from build123d import *

# Parameters (mm, degrees)
SKETCH1_R           = 15
BOSS_EXTRUDE1_DEPTH = 10
SKETCH2_R           = 22.5
BOSS_EXTRUDE2_DEPTH = 8
CHAMFER1_SIZE       = 1
SKETCH3_R           = 10
CUT_EXTRUDE1_DEPTH  = 10
CUT_EXTRUDE2_DEPTH  = 3
CHAMFER2_SIZE       = 1


with BuildPart() as part:
    # Sketch1 → Boss-Extrude1 (new body)
    with BuildSketch(Plane(origin=(0, 0, 0), x_dir=(1, 0, 0), z_dir=(0, 1, 0))):
        with Locations(Location((0, 0, 0), (0, 0, 270))):
            Circle(SKETCH1_R)
    extrude(amount=BOSS_EXTRUDE1_DEPTH)

    # Sketch2 → Boss-Extrude2 (add)
    with BuildSketch(Plane(origin=(0, 10, 0), x_dir=(1, 0, 0), z_dir=(0, 1, 0))):
        with Locations(Location((0, 0, 0), (0, 0, 270))):
            Circle(SKETCH2_R)
    extrude(amount=BOSS_EXTRUDE2_DEPTH)

    # Chamfer1
    chamfer1_edges = [part.edges().sort_by_distance(p)[0] for p in [
        (0, 0, -15),
    ]]
    chamfer(chamfer1_edges, length=CHAMFER1_SIZE)

    # Sketch3 → Cut-Extrude1 (cut)
    with BuildSketch(Plane.XZ):
        with Locations(Location((0, 0, 0), (0, 0, 270))):
            Circle(SKETCH3_R)
    extrude(amount=-CUT_EXTRUDE1_DEPTH, mode=Mode.SUBTRACT)

    # Sketch4 → Cut-Extrude2 (cut)
    with BuildSketch(Plane(origin=(0, 18, 0), x_dir=(1, 0, 0), z_dir=(0, 1, 0))):
        Polygon((5.326189108, -2.228237625), (4.592804943, 3.49849626), (-0.733384165, 5.726733886), (-5.326189108, 2.228237625), (-4.592804943, -3.49849626), (0.733384165, -5.726733886), align=None)
    extrude(amount=-CUT_EXTRUDE2_DEPTH, mode=Mode.SUBTRACT)

    # Chamfer2
    chamfer2_edges = [part.edges().sort_by_distance(p)[0] for p in [
        (0, 0, 10),
    ]]
    chamfer(chamfer2_edges, length=CHAMFER2_SIZE)


solid = part.part
Check sheet for the modelled part. Datum: model origin and axes. Units: mm. A direction names the side the tool comes from. Coordinates: 2 decimals unless noted, no trailing zeros. Loops run counter-clockwise (first coordinate to the right, second up) from the corner with the lowest first, then second, coordinate; pieces in that order, holes last. Notation, with made-up numbers: (-24.75, 32.25) -> (5.25, 32.25) arc R27 cw to (5.25, 58.25) -> close; hole circle Ø10 at (-13.75, 10). An arc over 180 degrees is marked (long way). Write item = value, one per line. Start each with the question number.
1. Draft check along X on faces 4 (the cylindrical face through (0.66, 5.437, -14.985)), 5 (the flat face through (4.965, 16.521, -0.595)), 6 (the flat face through (-4.965, 16.521, 0.595)), 7 (the flat face through (-5, 10, 15)). Enter one of: released by +X, released by -X, zero draft, split by the parting line, or undercut.
2. Section check D-D on z = 17.5. Record the cut outline in (x, y).
3. Section check A-A on y = 8.5. Record the cut outline in (x, z), then the cut area to 3 significant figures.
4. Depth check by flat-ended pin: P1, Ø10, axis at y = 7.5, z = 6, coming from the +X side; P2, Ø3, axis at x = 3.5, z = 6.5, coming from the -Y side; P3, Ø3, axis at x = -14, y = 6, coming from the +Z side. Enter the tip coordinate at first touch or a pass-through.
5. Section check C-C on z = 0. Record the cut outline in (x, y), then the cut area to 3 significant figures.
6. Material ranges on line 1 (Z direction, x = -0.5, y = 9.5); line 2 (X direction, y = 3, z = 0); line 3 (Y direction, x = 9, z = -4), recorded low to high.
7. Tool access check on faces 1 (the flat face through (0, 10, 0)), 2 (the flat face through (-9.3, 0, 6.2)), 3 (the flat face through (3, 17, 4)). Record the directions out of +Z, -Z, +X, -X, +Y, -Y that give a thin tool (end or side, any length) a straight path to the whole face; none if there is none.
8. Section check B-B on x = 0. Record the cut outline in (y, z).
Responses:
q1.face_4 = split by the parting line
q1.face_5 = undercut
q1.face_6 = undercut
q1.face_7 = zero draft
q2.outline = (-14.14, 10) -> (14.14, 10) -> (14.14, 18) -> (-14.14, 18) -> close
q3.outline = circle Ø30 at (0, 0); hole circle Ø20 at (0, 0)
q3.area = 393 mm2
q4.P1 = 22.44
q4.P2 = 10
q4.P3 = 8.29
q5.outline = (-22.5, 10) -> (-15, 10) -> (-15, 1) -> (-14, 0) -> (-11, 0) -> (-10, 1) -> (-10, 10) -> (10, 10) -> (10, 1) -> (11, 0) -> (14, 0) -> (15, 1) -> (15, 10) -> (22.5, 10) -> (22.5, 18) -> (5.04, 18) -> (5.04, 15) -> (-5.04, 15) -> (-5.04, 18) -> (-22.5, 18) -> close
q5.area = 428 mm2
q6.line_1 = -14.99 to -9.99, 9.99 to 14.99
q6.line_2 = -15 to -10, 10 to 15
q6.line_3 = 10 to 18
q7.face_1 = -Y
q7.face_2 = +Z, -Z, +X, -X, -Y
q7.face_3 = +Y
q8.outline = (0, -14) -> (1, -15) -> (10, -15) -> (10, -22.5) -> (18, -22.5) -> (18, -5.42) -> (15, -5.42) -> (15, 5.42) -> (18, 5.42) -> (18, 22.5) -> (10, 22.5) -> (10, 15) -> (1, 15) -> (0, 14) -> (0, 11) -> (1, 10) -> (10, 10) -> (10, -10) -> (1, -10) -> (0, -11) -> close
